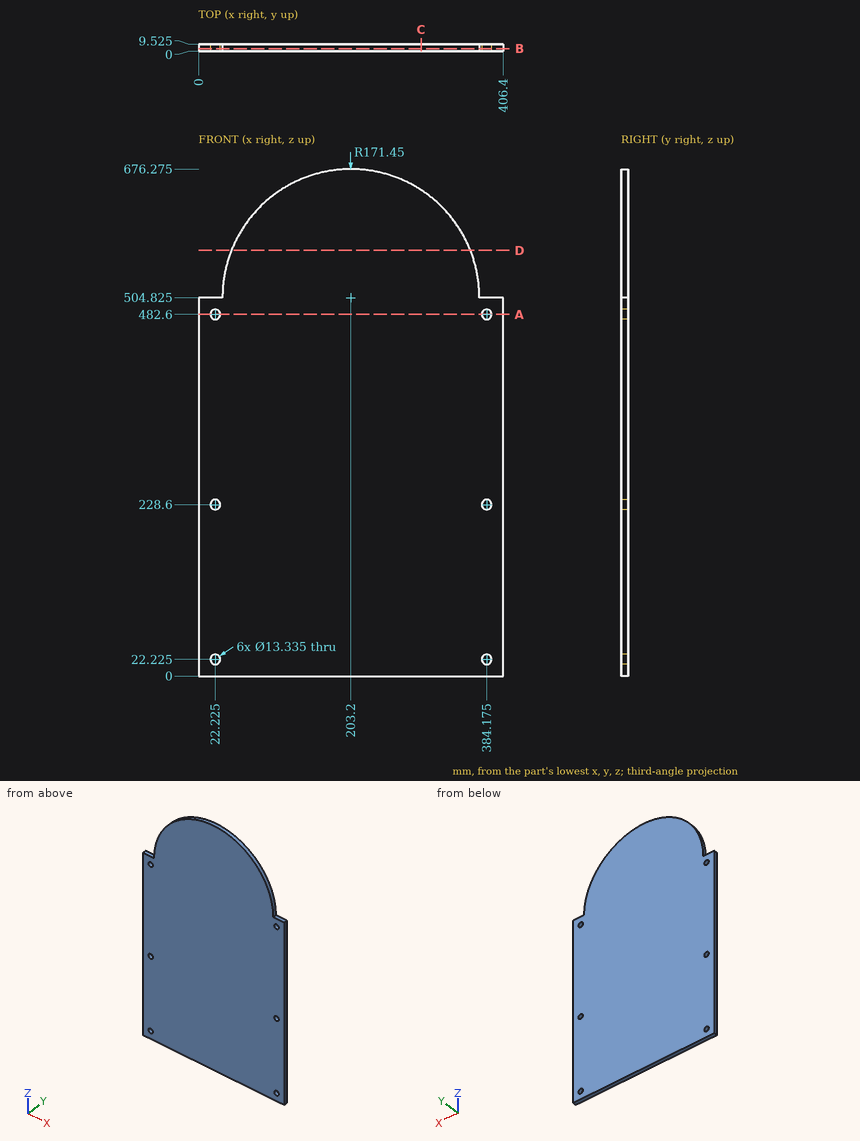
Verification items for this drawing (mm, ordinates from the low corner). Coordinates: 2 decimals unless noted, no trailing zeros. Order: outer loops, then holes, each group sorted by start corner. A loop starts at its lowest first (then second) coordinate and runs counter-clockwise, first axis right, second up. Notation, with made-up numbers: M 82.5,74.5 L 134.5,74.5 A14 cw 134.5,87.5 Z; hole C 17.5,45.5 d2. An arc over 180 degrees is marked long. Use CSV: the item, a comma, the result in double quotes.
Item 1: Cross-section at D-D on z = 568. Record the cut outline in (x, y) (3 decimals), then the cut area to 3 significant figures.
Returned:
outline,"M 43.814,0 L 362.586,0 L 362.586,9.525 L 43.814,9.525 Z"
area,"3,040 mm2"
Item 2: Cross-section at C-C on x = 297. Record the cut outline in (y, z) (3 decimals), then the cut area to 3 significant figures.
Returned:
outline,"M 0,0 L 9.525,0 L 9.525,648.34 L 0,648.34 Z"
area,"6,180 mm2"
Item 3: Cross-section at A-A on z = 482.6. Record the cut outline in (x, y) (1 decimal).
Returned:
outline,"M 0,0 L 15.6,0 L 15.6,9.5 L 0,9.5 Z; M 28.9,0 L 377.5,0 L 377.5,9.5 L 28.9,9.5 Z; M 390.8,0 L 406.4,0 L 406.4,9.5 L 390.8,9.5 Z"
Item 4: Gauge pin test, flat ends, axial feed: pin 1 Ø10.5 at (x, z) = (22.225, 482.6) entering from +Y; pin 2 Ø1.5 at (x, y) = (182.5, 8) entering from +Z; pin 3 Ø5 at (x, y) = (387.5, 3.5) entering from +Z (3 decimals). Record the tip position at first contact, or that the pin passes through.
Returned:
pin 1,"passes through"
pin 2,"stops at z = 675.11"
pin 3,"stops at z = 504.825"
Item 5: Thickness scan on line 1 along X through (y, z) = (5.5, 228.6); line 2 along Z through (x, y) = (198.5, 8.5); line 3 along Z through (x, y) = (209.5, 3.5). Record the ranges inside material, lowest first.
Returned:
line 1,"x = 0 to 15.56, 28.89 to 377.51, 390.84 to 406.4"
line 2,"z = 0 to 676.21"
line 3,"z = 0 to 676.16"
Item 6: Cross-section at B-B on y = 3.25. Give the number of separate pieces and of enclosed holes in the cut face, then the cut area to 3 significant figures.
Returned:
separate pieces,"1"
enclosed holes,"6"
area,"250,000 mm2"
